Can you work these out from the model? Positions are in its coordinate system, mm. Round coordinates to 2 decimals unless told otherwise and drop trailing zeros. Write each loop counter-clockwise with the first axis right and the second up, starting at its lowest first coordinate (ties: lowest second). Pieces come first, ordered by that corner, then holes. Notation, with made-up numbers: M 54.5,-11.75 L 61.5,-11.75 A12 ccw 61.5,8.25 Z; hole C 53.25,63.5 d10. An arc over 180 degrees is marked long. Answer in a Markdown table with one row per item. Add a question column.
(1) Suppose I cut it at D-D, the plane x = 165.1. Write out the boundary of the cut face in (y, z), then the cut area to 3 significant figures.
(2) Suppose I cut it at B-B, the plane y = 0. Write out the boundary of the cut face in (x, z).
(3) If I drill on probe 1 along Y at (x, z) = (0, 8); probe 2 along Y at (x, z) = (-166, 10); probe 3 along Y at (x, z) = (159, 11), over which ranges is the centre line in solid material (lowest first)?
(4) I'm going to push a flat-ended pin straight in: pin 1 (12.5 mm diameter, centred on x = 165.1, y = 0, fed in from -Z). Where does the tip first touch, or does it pass through?
(5) Suppose I cut it at A-A, the plane x = 0. Write out the boundary of the cut face in (y, z), then the cut area to 3 significant figures.
(6) If we mould it in two halves opening along X, with no side actions, what happens to faces 1 (the face through (-2.24, -175.18, 6.44)), 2 (the face through (-203.2, -3, 6)), 3 (the face through (203.2, -3, 6)), 4 (the face through (9.85, 168.2, 6.44))? For each: released by +X, released by -X, zero draft, split by the parting line, or undercut.
(7) Suppose I cut it at C-C, the plane y = -165.1. Write out the boundary of the cut face in (x, z).
from build123d import *

# Parameters (mm, degrees)
F0_W     = 406.4
F0_H     = 406.4
F1_DEPTH = 12.7
F2_R     = 10.3251
F3_DEPTH = 25.4


with BuildPart() as f1:
    # F0 (on Top) → F1 (new body)
    with BuildSketch(Plane.XY):
        Rectangle(F0_W, F0_H)
    extrude(amount=F1_DEPTH)

    # F2 (on face) → F3 (cut)
    with BuildSketch(Plane.XY.offset(12.7)):
        with Locations((-164.984982, 165.1)):
            Circle(F2_R)
        with Locations((-166.304624, 50.8)):
            Circle(F2_R)
        with Locations((-166.304624, -50.8)):
            Circle(F2_R)
        with Locations((-164.984982, -165.1)):
            Circle(F2_R)
        with Locations((164.984982, 165.1)):
            Circle(F2_R)
        with Locations((164.984982, -165.1)):
            Circle(F2_R)
        with Locations((165.1, 0)):
            Circle(F2_R)
        with Locations((0, 165.1)):
            Circle(F2_R)
        with Locations((0, -165.1)):
            Circle(F2_R)
    extrude(amount=-F3_DEPTH, mode=Mode.SUBTRACT)


solid = f1.part
Calculated:
| question | item | result |
|---|---|---|
| 1 | outline | M -203.2,0 L -175.42,0 L -175.42,12.7 L -203.2,12.7 Z; M -154.78,0 L -10.33,0 L -10.33,12.7 L -154.78,12.7 Z; M 10.33,0 L 154.78,0 L 154.78,12.7 L 10.33,12.7 Z; M 175.42,0 L 203.2,0 L 203.2,12.7 L 175.42,12.7 Z |
| 1 | area | 4,370 mm² |
| 2 | outline | M -203.2,0 L 154.77,0 L 154.77,12.7 L -203.2,12.7 Z; M 175.43,0 L 203.2,0 L 203.2,12.7 L 175.43,12.7 Z |
| 3 | probe 1 | -203.2 to -175.43, -154.77 to 154.77, 175.43 to 203.2 |
| 3 | probe 2 | -203.2 to -175.38, -154.82 to -61.12, -40.48 to 40.48, 61.12 to 154.82, 175.38 to 203.2 |
| 3 | probe 3 | -203.2 to -173.51, -156.69 to -8.33, 8.33 to 156.69, 173.51 to 203.2 |
| 4 | pin 1 | through |
| 5 | outline | M -203.2,0 L -175.43,0 L -175.43,12.7 L -203.2,12.7 Z; M -154.77,0 L 154.77,0 L 154.77,12.7 L -154.77,12.7 Z; M 175.43,0 L 203.2,0 L 203.2,12.7 L 175.43,12.7 Z |
| 5 | area | 4,640 mm² |
| 6 | face 1 | undercut |
| 6 | face 2 | released by -X |
| 6 | face 3 | released by +X |
| 6 | face 4 | undercut |
| 7 | outline | M -203.2,0 L -175.31,0 L -175.31,12.7 L -203.2,12.7 Z; M -154.66,0 L -10.33,0 L -10.33,12.7 L -154.66,12.7 Z; M 10.33,0 L 154.66,0 L 154.66,12.7 L 10.33,12.7 Z; M 175.31,0 L 203.2,0 L 203.2,12.7 L 175.31,12.7 Z |
